Autodesk Inventor part; units mm, degrees
ref_plane "YZ Plane" through (0, 0, 0) normal (1, 0, 0) x (0, 1, 0)
ref_plane "XZ Plane" through (0, 0, 0) normal (0, 1, 0) x (-1, 0, 0)
ref_plane "XY Plane" through (0, 0, 0) normal (0, 0, 1) x (1, 0, 0)
sketch "Sketch1" plane through (0, 0, 0) normal (0, 1, 0) x (-1, 0, 0)
  line L0 (15.5, 15.5) -> (-15.5, 15.5)
  line L1 (-15.5, 15.5) -> (-15.5, -15.5)
  line L2 (-15.5, -15.5) -> (15.5, -15.5)
  line L3 (15.5, -15.5) -> (15.5, 15.5)
  line L4 (15.5, 15.5) -> (-15.5, -15.5) construction
  line L5 (-15.5, 15.5) -> (15.5, -15.5) construction
  line L6 (21, 21) -> (-21, 21)
  line L7 (-21, 21) -> (-21, -21)
  line L8 (-21, -21) -> (21, -21)
  line L9 (21, -21) -> (21, 21)
  line L10 (21, 21) -> (-21, -21) construction
  line L11 (-21, 21) -> (21, -21) construction
  line L12 (24, 26) -> (-24, 26)
  line L13 (-26, 24) -> (-26, -24)
  line L14 (-24, -26) -> (24, -26)
  line L15 (26, -24) -> (26, 24)
  circle A0 centre (0, 0) radius 2.5
  arc A1 (26, 24) -> (24, 26) centre (24, 24) ccw
  arc A2 (-24, 26) -> (-26, 24) centre (-24, 24) ccw
  arc A3 (24, -26) -> (26, -24) centre (24, -24) ccw
  arc A4 (-26, -24) -> (-24, -26) centre (-24, -24) ccw
  point P0 (26, 26)
  point P1 (-26, 26)
  point P2 (-26, -26)
  point P3 (26, -26)
  dimension "d0" = 31
  dimension "d1" = 31
  dimension "d2" = 42
  dimension "d3" = 42
  dimension "d4" = 5
  dimension "d7" = 5
  dimension "d23" = 2
extrude "Extrusion1" add sketch "Sketch1" against normal blind 2 contours L3 L2 L1 L0 | L9 L8 L7 L6 | A0
extrude "Extrusion2" add sketch "Sketch1" against normal blind 30 contours A1 L15 A3 L14 A4 L13 A2 L12
hole "Hole1" at (-15.5, 0, -15.5) at (-15.5, 0, 15.5) at (15.5, 0, 15.5) at (15.5, 0, -15.5) direction (0, -1, 0) diameter 2.45 end through all
thread "Thread2"
extrude "Extrusion3" cut sketch "Sketch1" against normal up to surface (2 mm away) contours A0
properties part number "turnmotorcasing"
Geometry check sheet. Reference: the model listing, model coordinates, mm. A direction names the side the tool comes from. Give positions to 0.01 mm unless a question says otherwise; leave off trailing zeros. Order: outer loops, then holes, each group sorted by start corner. A loop starts at its lowest first (then second) coordinate and runs counter-clockwise, first axis right, second up. Notation, with made-up numbers: (50, 28.5) - (88, 28.5) arc R32 ccw to (88, 55.5) - close; hole circle Ø1 at (1, -13.75). An arc over 180 degrees is marked (long way). Write item = value, one per line. Start each with the question number.
1) Section check B-B (y = -7.25). Enter the section's corners in (x, z).
2) Section check C-C (x = 15.5). Enter the section's corners in (y, z) (3 decimals), then the cut area to 3 significant figures.
3) Gauge pin test, flat ends, axial feed: pin 1 Ø2 at (x, z) = (-15.5, -15.5) entering from +Y; pin 2 Ø10 at (x, z) = (10.5, -7.5) entering from -Y. Record the tip position at first contact, or that the pin passes through.
4) Access from +Z, -Z, +X, -X, +Y, -Y to the whole of each face (thin tool, end or side, straight path). Record for faces 1 (the flat face through (0, -16, 21)), 2 (the cylindrical face through (0.54, -0.99, -2.44)).
5) Section check D-D (z = 0). Enter the section's corners in (x, y).
6) Scan lines: L1, parallel to X at y = -1.4, z = -15.5 (3 decimals); L2, parallel to X at y = -22.25, z = 17.5. Record each from-to range of solid material in increasing order.
7) Draft check along Z on faces 3 (the cylindrical face through (-25.43, -14.79, 25.4)), 4 (the flat face through (0, -15, -26)), 5 (the flat face through (-21, -16, 0)). Enter one of: released by +Z, released by -Z, zero draft, split by the parting line, or undercut.
8) Section check A-A (z = -15.5). Enter the section's corners in (x, y) (3 decimals).
Geometry check:
q1.outline = (-26, -24) arc R2 ccw to (-24, -26) - (24, -26) arc R2 ccw to (26, -24) - (26, 24) arc R2 ccw to (24, 26) - (-24, 26) arc R2 ccw to (-26, 24) - close; hole (-21, -21) - (21, -21) - (21, 21) - (-21, 21) - close
q2.outline = (-30, -26) - (0, -26) - (0, -16.725) - (-2, -16.725) - (-2, -21) - (-30, -21) - close; (-30, 21) - (-2, 21) - (-2, 16.725) - (0, 16.725) - (0, 26) - (-30, 26) - close; (-2, -14.275) - (0, -14.275) - (0, 14.275) - (-2, 14.275) - close
q2.area = 374 mm2
q3.pin_1 = through
q3.pin_2 = -2
q4.face_1 = -Y
q4.face_2 = +Y, -Y
q5.outline = (-26, -30) - (-21, -30) - (-21, -2) - (-2.5, -2) - (-2.5, 0) - (-26, 0) - close; (2.5, -2) - (21, -2) - (21, -30) - (26, -30) - (26, 0) - (2.5, 0) - close
q6.L1 = -26 to -16.725, -14.275 to 14.275, 16.725 to 26
q6.L2 = -26 to -21, 21 to 26
q7.face_3 = released by +Z
q7.face_4 = released by -Z
q7.face_5 = undercut
q8.outline = (-26, -30) - (-21, -30) - (-21, -2) - (-16.725, -2) - (-16.725, 0) - (-26, 0) - close; (-14.275, -2) - (14.275, -2) - (14.275, 0) - (-14.275, 0) - close; (16.725, -2) - (21, -2) - (21, -30) - (26, -30) - (26, 0) - (16.725, 0) - close
